```python
from build123d import *

# Parameters (mm, degrees)
F1_DEPTH  = 112.014
F3_DEPTH  = 17.272
F4_R      = 3.3623176789
F5_DEPTH  = 25.4
F6_R      = 3.1543384868
F7_DEPTH  = 25.4
F8_W      = 38.0456186831
F8_H      = 21.038826555
F9_DEPTH  = 25.4
F10_DEPTH = 8.382
F11_DEPTH = 10.414
F12_DEPTH = 9.652
F13_DEPTH = 11.684
F14_R     = 3.9810308691
F14_R_2   = 3.9967217836
F15_DEPTH = 25.4


with BuildPart() as f1:
    # F0 (on Top) → F1 (new body)
    with BuildSketch(Plane.XY):
        with BuildLine():
            ThreePointArc((-94.7144221793, 78.996181488), (-97.4408484509, 37.4965810895), (-77.4463454997, 1.029197235))
            ThreePointArc((-77.4463454997, 1.029197235), (-82.0851675961, -39.9590099953), (-40.8864470189, -42.0125983655))
            Line((-40.8864470189, -42.0125983655), (-3.1338073313, -42.0125983655))
            Line((-3.1338073313, -42.0125983655), (-3.1338073313, -28.7388270008))
            ThreePointArc((-3.1338073313, -28.7388270008), (7.6465004578, -22.6188809922), (14.1175022251, -12.0455697179))
            Line((14.1175022251, -12.0455697179), (59.5423281193, -12.0455697179))
            Line((59.5423281193, -12.0455697179), (59.5423281193, 20.0759489089))
            Line((59.5423281193, 20.0759489089), (41.4761226971, 20.0759489089))
            ThreePointArc((41.4761226971, 20.0759489089), (32.6284517751, 100.6595778454), (-44.6295377394, 125.2198219299))
            Line((-44.6295377394, 125.2198219299), (-110.9817028046, 125.2198219299))
            Line((-110.9817028046, 125.2198219299), (-110.9817028046, 78.996181488))
            Line((-110.9817028046, 78.996181488), (-94.7144221793, 78.996181488))
        make_face()
    extrude(amount=F1_DEPTH)

    # F2 (on face) → F3 (join)
    with BuildSketch(Plane.XY.offset(112.014)):
        Polygon((-34.9643416703, 80.2690163255), (-57.5213618577, 81.0558870435), (-57.5213618577, 62.1709451079), (-34.9643416703, 62.1709451079), align=None)
    extrude(amount=F3_DEPTH)

    # F4 (on face) → F5 (join)
    with BuildSketch(Plane(origin=(2.7541761254, 78.9532575536, 0), x_dir=(-0.9993921209, 0.0348624237, 0), z_dir=(0.0348624237, 0.9993921209, 0))):
        with Locations((42.88270697, 122.0109984279)):
            Circle(F4_R)
    extrude(amount=F5_DEPTH)

    # F6 (on face) → F7 (join)
    with BuildSketch(Plane(origin=(2.7541761254, 78.9532575536, 0), x_dir=(-0.9993921209, 0.0348624237, 0), z_dir=(0.0348624237, 0.9993921209, 0))):
        with Locations((55.5666647851, 120.65)):
            Circle(F6_R)
    extrude(amount=F7_DEPTH)

    # F8 (on face) → F9 (join)
    with BuildSketch(Plane.XY.offset(112.014)):
        with Locations((-0.6137024611, 72.2188074142)):
            Rectangle(F8_W, F8_H)
    extrude(amount=F9_DEPTH)

    # F10 (add): a face of the model
    f10_faces = [f1.faces().sort_by_distance(p)[0] for p in [
        (-0.6137024611, 72.2188074142, 137.414),
    ]]
    extrude(f10_faces, amount=-F10_DEPTH)

    # F11 (add): a face of the model
    f11_faces = [f1.faces().sort_by_distance(p)[0] for p in [
        (-0.6137024611, 72.2188074142, 137.414),
    ]]
    extrude(f11_faces, amount=-F11_DEPTH)

    # F12 (add): a face of the model
    f12_faces = [f1.faces().sort_by_distance(p)[0] for p in [
        (-0.6137024611, 72.2188074142, 137.414),
    ]]
    extrude(f12_faces, amount=-F12_DEPTH)

    # F13 (add): a face of the model
    f13_faces = [f1.faces().sort_by_distance(p)[0] for p in [
        (-0.6137024611, 72.2188074142, 137.414),
    ]]
    extrude(f13_faces, amount=-F13_DEPTH)

    # F14 (on face) → F15 (join)
    with BuildSketch(Plane(origin=(0, 82.7382206917, 0), x_dir=(-1, 0, 0), z_dir=(0, 1, 0))):
        with Locations((-10.8387600631, 126.1480897665)):
            Circle(F14_R)
        with Locations((9.6803465858, 126.1480897665)):
            Circle(F14_R_2)
    extrude(amount=F15_DEPTH)


solid = f1.part
```
Work out the finished part from the listing and answer in its coordinate system (mm). A direction names the side the tool comes from. Coordinates: 2 decimals unless noted, no trailing zeros. Loops run counter-clockwise (first coordinate to the right, second up) from the corner with the lowest first, then second, coordinate; pieces in that order, holes last. Notation, with made-up numbers: (63, -23) - (84, -23) arc R19 cw to (84, -3) - close; hole circle Ø11 at (14, 31.5). An arc over 180 degrees is marked (long way). Use a Markdown table: item, result.
Item 1: Consider probe 1 along X at (y, z) = (63, 122); probe 2 along Z at (x, y) = (19, 1); probe 3 along Y at (x, z) = (-86.5, 11). Determine where each line is inside the solid, lowest interval first. Write a range as from..to.
Evaluation:
| item | result |
|---|---|
| probe 1 | x = -57.52..-34.96, -19.64..18.41 |
| probe 2 | z = 0..112.01 |
| probe 3 | y = -32.85..-10.44, 12.02..125.22 |
Item 2: Find section C-C, the plane y = 33. Determine the outline of the cut face in (x, z), and give its area (3 significant figures).
Evaluation:
| item | result |
|---|---|
| outline | (-96.3, 0) - (46.55, 0) - (46.55, 112.01) - (-96.3, 112.01) - close |
| area | 16,000 mm2 |
Item 3: Find section A-A, the plane z = 27.5. Determine the outline of the cut face in (x, y), and give its area (3 significant figures).
Evaluation:
| item | result |
|---|---|
| outline | (-110.98, 79) - (-94.71, 79) arc R74.32 ccw to (-77.45, 1.03) arc R28.29 ccw (long way) to (-40.89, -42.01) - (-3.13, -42.01) - (-3.13, -28.74) arc R24.8 ccw to (14.12, -12.05) - (59.54, -12.05) - (59.54, 20.08) - (41.48, 20.08) arc R74.32 ccw to (-44.63, 125.22) - (-110.98, 125.22) - close |
| area | 22,500 mm2 |
Item 4: Find section D-D, the plane x = 33.5. Determine the outline of the cut face in (y, z).
Evaluation:
| item | result |
|---|---|
| outline | (-12.05, 0) - (99.57, 0) - (99.57, 112.01) - (-12.05, 112.01) - close |
Item 5: The mould has two halves that part along X. Classify faces 6 (the flat face through (18.409, 72, 125)), 7 (the flat face through (-1, 72, 137.414)), 8 (the cylindrical face through (-38.94, 92.94, 118.73)): +X half, -X half, draft (parallel to the pull), parting line (faces both ways), or undercut.
Evaluation:
| item | result |
|---|---|
| face 6 | +X half |
| face 7 | draft |
| face 8 | undercut |
Item 6: Given pin 1 Ø1.5 at (x, z) = (39, 108) entering from -Y; pin 2 Ø21 at (x, y) = (-45.5, 73) entering from +Z; pin 3 Ø6.5 at (y, z) = (76.5, 118.5) entering from +X, each flat-ended and moving along its own axis, determine where each tip first touches the part or whether it passes through.
Evaluation:
| item | result |
|---|---|
| pin 1 | stops at y = -12.05 |
| pin 2 | stops at z = 129.29 |
| pin 3 | stops at x = 18.41 |
Item 7: For faces 1 (the cylindrical face through (-11.52, 95.26, 122.6)), 2 (the flat face through (-77, 125.22, 55)), 3 (the flat face through (-1, 61.699, 125)), 4 (the flat face through (-3.134, -35, 55)), 5 (the flat face through (-57.521, 72, 121)), determine the directions among +Z, -Z, +X, -X, +Y, -Y from which every point of the face is accessible in a straight line to the end or side of a thin tool.
Evaluation:
| item | result |
|---|---|
| face 1 | +Y |
| face 2 | +Z, -Z, -X, +Y |
| face 3 | +Z, +X, -X, -Y |
| face 4 | +Z, -Z, +X, -Y |
| face 5 | +Z, -X, +Y, -Y |
Item 8: Find section B-B, the plane x = -8.5. Determine the outline of the cut face in (y, z).
Evaluation:
| item | result |
|---|---|
| outline | (-42.01, 0) - (126.07, 0) - (126.07, 112.01) - (82.74, 112.01) - (82.74, 122.33) - (108.14, 122.33) - (108.14, 129.97) - (82.74, 129.97) - (82.74, 137.41) - (61.7, 137.41) - (61.7, 112.01) - (-42.01, 112.01) - close |
